Could you check a few things on this model? Use its own coordinates, in mm. Face numbers are marked on the shaded views. A direction names the side the tool comes from. Give positions to 0.01 mm unless a question says otherwise; leave off trailing zeros. Order: outer loops, then holes, each group sorted by start corner. A loop starts at its lowest first (then second) coordinate and runs counter-clockwise, first axis right, second up.
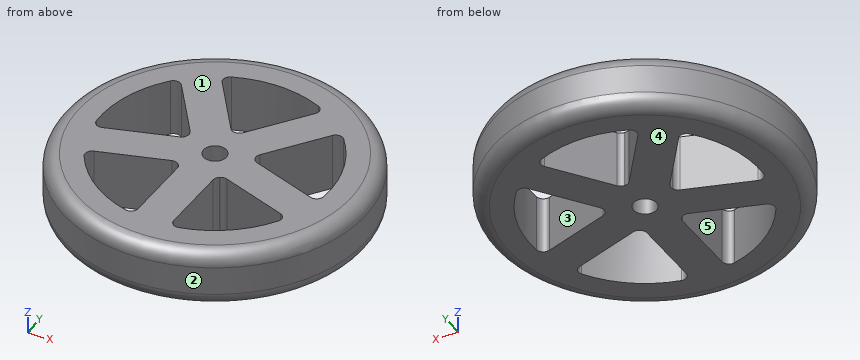
from build123d import *

# Parameters (mm, degrees)
ESQUISSE1_R                  = 105
BOSS_EXTRU_1_DEPTH           = 40
ENL_V_MAT_EXTRU_1_DEPTH      = 154.785564992
ENL_V_MAT_EXTRU_1_DEPTH_BACK = 154.785564992
ENL_V_MAT_EXTRU_2_DEPTH      = 154.785564992
ENL_V_MAT_EXTRU_2_DEPTH_BACK = 154.785564992
ESQUISSE3_R                  = 8
CONG_1_R                     = 5
CONG_2_R                     = 10


with BuildPart() as part:
    # Esquisse1 → Boss.-Extru.1 (new body)
    with BuildSketch(Plane.XY):
        Circle(ESQUISSE1_R)
    extrude(amount=BOSS_EXTRU_1_DEPTH)

    # Esquisse2 → Enlèv. mat.-Extru.1 (cut, two sides: drawn at the far end of the back side and taken through both)
    with BuildSketch(Plane.XY.offset(40).offset(-ENL_V_MAT_EXTRU_1_DEPTH_BACK)):
        with BuildLine():
            Line((2.613211582, 24.863047384), (36.332551814, 71.27373765))
            ThreePointArc((36.332551814, 71.27373765), (0, 80), (-36.332551814, 71.27373765))
            Line((-36.332551814, 71.27373765), (-2.613211582, 24.863047384))
            ThreePointArc((-2.613211582, 24.863047384), (0, 25), (2.613211582, 24.863047384))
        make_face()
        with BuildLine():
            Line((24.453690018, 5.19779227), (79.012728593, -12.52951397))
            ThreePointArc((79.012728593, -12.52951397), (76.084521304, 24.72135955), (56.557976674, 56.579106343))
            Line((56.557976674, 56.579106343), (22.838636441, 10.168416077))
            ThreePointArc((22.838636441, 10.168416077), (23.776412907, 7.725424859), (24.453690018, 5.19779227))
        make_face()
        with BuildLine():
            Line((12.5, -21.650635095), (12.5, -79.017403146))
            ThreePointArc((12.5, -79.017403146), (47.022820183, -64.72135955), (71.287303733, -36.305926877))
            Line((71.287303733, -36.305926877), (16.728265159, -18.578620637))
            ThreePointArc((16.728265159, -18.578620637), (14.694631307, -20.225424859), (12.5, -21.650635095))
        make_face()
        with BuildLine():
            Line((-16.728265159, -18.578620637), (-71.287303733, -36.305926877))
            ThreePointArc((-71.287303733, -36.305926877), (-47.022820183, -64.72135955), (-12.5, -79.017403146))
            Line((-12.5, -79.017403146), (-12.5, -21.650635095))
            ThreePointArc((-12.5, -21.650635095), (-14.694631307, -20.225424859), (-16.728265159, -18.578620637))
        make_face()
        with BuildLine():
            Line((-22.838636441, 10.168416077), (-56.557976674, 56.579106343))
            ThreePointArc((-56.557976674, 56.579106343), (-76.084521304, 24.72135955), (-79.012728593, -12.52951397))
            Line((-79.012728593, -12.52951397), (-24.453690018, 5.19779227))
            ThreePointArc((-24.453690018, 5.19779227), (-23.776412907, 7.725424859), (-22.838636441, 10.168416077))
        make_face()
    extrude(amount=ENL_V_MAT_EXTRU_1_DEPTH + ENL_V_MAT_EXTRU_1_DEPTH_BACK, mode=Mode.SUBTRACT)

    # Esquisse3 → Enlèv. mat.-Extru.2 (cut, two sides: drawn at the far end of the back side and taken through both)
    with BuildSketch(Plane.XY.offset(40).offset(-ENL_V_MAT_EXTRU_2_DEPTH_BACK)):
        Circle(ESQUISSE3_R)
    extrude(amount=ENL_V_MAT_EXTRU_2_DEPTH + ENL_V_MAT_EXTRU_2_DEPTH_BACK, mode=Mode.SUBTRACT)

    # Congé1
    cong_1_edges = [part.edges().sort_by_distance(p)[0] for p in [
        (-79.012728593, -12.52951397, 20),
        (-56.557976674, 56.579106343, 20),
        (-22.838636441, 10.168416077, 20),
        (-24.453690018, 5.19779227, 20),
        (-12.5, -79.017403146, 20),
        (-71.287303733, -36.305926877, 20),
        (-16.728265159, -18.578620637, 20),
        (-12.5, -21.650635095, 20),
        (71.287303733, -36.305926877, 20),
        (12.5, -79.017403146, 20),
        (12.5, -21.650635095, 20),
        (16.728265159, -18.578620637, 20),
        (56.557976674, 56.579106343, 20),
        (79.012728593, -12.52951397, 20),
        (24.453690018, 5.19779227, 20),
        (22.838636441, 10.168416077, 20),
        (-36.332551814, 71.27373765, 20),
        (36.332551814, 71.27373765, 20),
        (2.613211582, 24.863047384, 20),
        (-2.613211582, 24.863047384, 20),
    ]]
    fillet(cong_1_edges, radius=CONG_1_R)

    # Congé2
    cong_2_edges = [part.edges().sort_by_distance(p)[0] for p in [
        (-105, 0, 0),
        (-105, 0, 40),
    ]]
    fillet(cong_2_edges, radius=CONG_2_R)


solid = part.part
Item 1: For the marked faces 4 and 5, which set-ups out of +Z, -Z, +X, -X, +Y, -Y let a thin tool reach every point of the face, with its end or its side?
Findings:
face 4: -Z, +X, -X, +Y, -Y
face 5: +Z, -Z
Item 2: Imagine slicing it at A-A on y = 0. List the corners of the cut face in (x, z) for me, then the cut area to 3 significant figures.
Findings:
outline: (-105, 10) arc R10 ccw to (-95, 0) - (-80, 0) - (-80, 40) - (-95, 40) arc R10 ccw to (-105, 30) - close; (-40.45, 0) - (-8, 0) - (-8, 40) - (-40.45, 40) - close; (8, 0) - (40.45, 0) - (40.45, 40) - (8, 40) - close; (80, 0) - (95, 0) arc R10 ccw to (105, 10) - (105, 30) arc R10 ccw to (95, 40) - (80, 40) - close
area: 4,510 mm2
Item 3: Please list where these lines run through material, in increasing order: line 1 along Y through (x, z) = (0, 19); line 2 along X through (y, z) = (9, 32.5); line 3 along Y through (x, z) = (-41, 7).
Findings:
line 1: y = -105 to -8, 8 to 25, 80 to 105
line 2: x = -104.29 to -79.49, -23.5 to 23.5, 79.49 to 104.29
line 3: y = -96.16 to -68.69, -26.46 to -0.18, 35.17 to 96.16
Item 4: For pin 1 (1 mm diameter, centred on y = -35.5, z = 34, fed in from +X); pin 2 (6 mm diameter, centred on x = -23, z = 20.5, fed in from -Y); pin 3 (1.5 mm diameter, centred on x = 58.5, z = 23.5, fed in from +Y), each with a flat end and sliding along its axis, tell me the tip position at first contact or that it passes through.
Findings:
pin 1: stops at x = 98.21
pin 2: stops at y = -103.08
pin 3: stops at y = 87.69
Item 5: Imagine slicing it at B-B on z = 19. Give the number of separate pieces and of enclosed holes in the cut face, then the cut area to 3 significant figures.
Findings:
separate pieces: 1
enclosed holes: 6
area: 23,400 mm2
Item 6: We'd pull the mould along X, two halves only. Please class the marked faces 1, 2 and 3: +X half, -X half, draft (parallel to the pull), parting line (faces both ways), or undercut.
Findings:
face 1: draft
face 2: parting line
face 3: undercut
